```python
from build123d import *

# Parameters (mm, degrees)
SKETCH1_W           = 16.5
SKETCH1_H           = 11.5
SKETCH1_W_2         = 10.5
SKETCH1_H_2         = 5.5
BOSS_EXTRUDE1_DEPTH = 17
CUT_EXTRUDE1_REACH  = 28.334
SKETCH2_R           = 2.5
SKETCH3_W           = 16.5
SKETCH3_H           = 11.5
BOSS_EXTRUDE2_DEPTH = 3
BOSS_EXTRUDE3_START = -11
SKETCH4_W           = 21.75
SKETCH4_H           = 11
BOSS_EXTRUDE3_DEPTH = 4
CHAMFER1_SIZE       = 5
CHAMFER2_SIZE       = 3
SKETCH5_R           = 1.1
SKETCH5_W           = 3
SKETCH5_H           = 2.684
BOSS_EXTRUDE4_DEPTH = 7
BOSS_EXTRUDE5_DEPTH = 11
CUT_EXTRUDE2_REACH  = 41.144
SKETCH7_W           = 10.5
SKETCH7_H           = 1.5


with BuildPart() as part:
    # Sketch1 → Boss-Extrude1 (new body)
    with BuildSketch(Plane(origin=(0, 0, 0), x_dir=(1, 0, 0), z_dir=(0, 1, 0))):
        with Locations((8.25, 5.75)):
            Rectangle(SKETCH1_W, SKETCH1_H)
        with Locations((8.25, 5.75)):
            Rectangle(SKETCH1_W_2, SKETCH1_H_2, mode=Mode.SUBTRACT)
    extrude(amount=BOSS_EXTRUDE1_DEPTH)

    # Sketch2 → Cut-Extrude1 (cut, up to next)
    with BuildSketch(Plane(origin=(0, 0, -11.5), x_dir=(-1, 0, 0), z_dir=(0, 0, -1)), mode=Mode.PRIVATE) as cut_extrude1_sk1:
        with Locations((-8.25, 10.5)):
            Circle(SKETCH2_R)
    cut_extrude1_tool1 = extrude(cut_extrude1_sk1.sketch, amount=-CUT_EXTRUDE1_REACH, mode=Mode.PRIVATE) & part.part
    add(cut_extrude1_tool1.solids().sort_by_distance((8.25, 10.5, -11.5))[0], mode=Mode.SUBTRACT)

    # Sketch3 → Boss-Extrude2 (add)
    with BuildSketch(Plane(origin=(0, 17, 0), x_dir=(1, 0, 0), z_dir=(0, 1, 0))):
        with Locations((8.25, 5.75)):
            Rectangle(SKETCH3_W, SKETCH3_H)
    extrude(amount=BOSS_EXTRUDE2_DEPTH)

    # Sketch4 → Boss-Extrude3 (add)
    with BuildSketch(Plane(origin=(0, 20, 0), x_dir=(1, 0, 0), z_dir=(0, 1, 0)).offset(BOSS_EXTRUDE3_START)):
        with Locations((-10.875, -2.176)):
            Rectangle(SKETCH4_W, SKETCH4_H)
    extrude(amount=BOSS_EXTRUDE3_DEPTH)

    # Chamfer1
    chamfer1_edges = [part.edges().sort_by_distance(p)[0] for p in [
        (0, 11, 0),
        (0, 11, -3.324),
    ]]
    chamfer(chamfer1_edges, length=CHAMFER1_SIZE)

    # Chamfer2
    chamfer2_edges = [part.edges().sort_by_distance(p)[0] for p in [
        (0, 13, -4.162),
        (0, 9, -4.162),
        (2.5, 13, 0),
        (2.5, 9, 0),
    ]]
    chamfer(chamfer2_edges, length=CHAMFER2_SIZE)

    # Sketch5 → Boss-Extrude4 (add)
    with BuildSketch(Plane(origin=(0, 13, 0), x_dir=(1, 0, 0), z_dir=(0, 1, 0))):
        with Locations(Location((-19.15, -2.46, 0), (0, 0, 270))):
            Circle(SKETCH5_R)
        with Locations(Location((-9.5, -2.46, 0), (0, 0, 270))):
            Circle(SKETCH5_R)
        with Locations((-19.15, 1.982)):
            Rectangle(SKETCH5_W, SKETCH5_H)
        with Locations((-9.5, 1.982)):
            Rectangle(SKETCH5_W, SKETCH5_H)
    extrude(amount=BOSS_EXTRUDE4_DEPTH)

    # Sketch6 → Boss-Extrude5 (add)
    with BuildSketch(Plane.XY.offset(7.676)):
        Polygon((-21.75, 13), (-24.65, 13), (-24.65, 20), (-27.65, 20), (-27.65, 9), (-21.75, 9), align=None)
    extrude(amount=-BOSS_EXTRUDE5_DEPTH)

    # Sketch7 → Cut-Extrude2 (cut, up to next)
    with BuildSketch(Plane(origin=(0, 0, -11.5), x_dir=(-1, 0, 0), z_dir=(0, 0, -1)), mode=Mode.PRIVATE) as cut_extrude2_sk1:
        with Locations((-8.25, 16.25)):
            Rectangle(SKETCH7_W, SKETCH7_H)
    cut_extrude2_tool1 = extrude(cut_extrude2_sk1.sketch, amount=-CUT_EXTRUDE2_REACH, mode=Mode.PRIVATE) & part.part
    add(cut_extrude2_tool1.solids().sort_by_distance((8.25, 16.25, -11.5))[0], mode=Mode.SUBTRACT)


solid = part.part
```
The listing builds one solid part. Answer for the finished solid, in the listing's coordinates (mm). A direction names the side the tool comes from. Give positions to 0.01 mm unless a question says otherwise; leave off trailing zeros. Order: outer loops, then holes, each group sorted by start corner. A loop starts at its lowest first (then second) coordinate and runs counter-clockwise, first axis right, second up. Notation, with made-up numbers: (14.25, -35) -> (62.25, -35) arc R31 ccw to (62.25, -8) -> close; hole circle Ø5 at (-34.5, 39.25). An arc over 180 degrees is marked (long way). Answer as a JSON object with one key per item and string values. Group by question number.
Item 1: A tool of negligible diameter and unlimited length cuts with its end or side. For faces 1 (the flat face through (-17, 12, 7.676)), 2 (the cylindrical face through (-10.17, 16.45, 1.59)), 3 (the flat face through (1, 15, 1)), 4 (the flat face through (-20.65, 16, -2)), from which of +Z, -Z, +X, -X, +Y, -Y can it reach the whole face along a straight path? Write none if from no direction.
Item 2: Determine the mould class of faces 5 (the cylindrical face through (8.79, 8.06, -10.02)), 6 (the flat face through (8, 8, -3)), 7 (the flat face through (8, 17, -7)), 8 (the flat face through (1, 8, 2)) for opening direction Y: pulls with the +Y half, pulls with the -Y half, needs draft (parallel to the pull), parting line crosses it, or undercut.
Item 3: The part is cut by section B-B on x = 8.25. Write down the section's boundary in (y, z), and give its area (3 significant figures).
Item 4: The part is cut by section A-A on y = 10.5. Write down the section's boundary in (x, z).
Item 5: Consider L1, parallel to Y at x = 8.25, z = -10.55; L2, parallel to X at y = 3.5, z = -3.5; L3, parallel to Z at x = 9.5, y = 1.5. Determine where each line is inside the solid, lowest interval first. Write a range as from..to.
Item 6: Flat-ended cylindrical pins translate along their axes: pin 1 (10 mm diameter, centred on x = -15.5, y = 12.5, fed in from -Z); pin 2 (8 mm diameter, centred on x = 11, z = -9, fed in from -Y); pin 3 (3 mm diameter, centred on x = -14.5, y = 17, fed in from +Z); pin 4 (2.5 mm diameter, centred on x = -9, y = 17.5, fed in from +Z). Find the tip coordinate at first contact, or state that the pin passes through.
Item 7: The part is cut by section C-C on x = -9.5. Write down the section's boundary in (y, z).
Item 8: The part is cut by section D-D on z = 2.46. Write down the section's boundary in (x, y).
Result set:
{
 "1": {"face 1": "+Z, +X, -X, +Y, -Y", "face 2": "+Y", "face 3": "+Z, +X, +Y", "face 4": "+Z, -Z, +Y"},
 "2": {"face 5": "undercut", "face 6": "needs draft", "face 7": "undercut", "face 8": "pulls with the -Y half"},
 "3": {"outline": "(0, -11.5) -> (8, -11.5) -> (8, -8.5) -> (0, -8.5) -> close; (0, -3) -> (17, -3) -> (17, -11.5) -> (20, -11.5) -> (20, 0) -> (0, 0) -> close; (13, -11.5) -> (15.5, -11.5) -> (15.5, -8.5) -> (13, -8.5) -> close", "area": "117 mm²"},
 "4": {"outline": "(-27.65, -3.32) -> (-5, -3.32) -> (0, -8.32) -> (0, -11.5) -> (5.75, -11.5) -> (5.75, -8.5) -> (3, -8.5) -> (3, -3) -> (13.5, -3) -> (13.5, -8.5) -> (10.75, -8.5) -> (10.75, -11.5) -> (16.5, -11.5) -> (16.5, 0) -> (5, 0) -> (0, 5) -> (0, 7.68) -> (-27.65, 7.68) -> close"},
 "5": {"L1": "0..8, 13..15.5, 17..20", "L2": "0..3, 13.5..16.5", "L3": "-11.5..-8.5, -3..0"},
 "6": {"pin 1": "z = -3.32", "pin 2": "y = 0", "pin 3": "through", "pin 4": "z = 3.56"},
 "7": {"outline": "(9, -3.32) -> (20, -3.32) -> (20, -0.64) -> (13, -0.64) -> (13, 1.36) -> (20, 1.36) -> (20, 3.56) -> (13, 3.56) -> (13, 7.68) -> (9, 7.68) -> close"},
 "8": {"outline": "(-27.65, 9) -> (-3, 9) -> (-2.46, 8.46) -> (2.54, 8.46) -> (2.54, 13.54) -> (-2.46, 13.54) -> (-3, 13) -> (-8.4, 13) -> (-8.4, 20) -> (-10.6, 20) -> (-10.6, 13) -> (-18.05, 13) -> (-18.05, 20) -> (-20.25, 20) -> (-20.25, 13) -> (-24.65, 13) -> (-24.65, 20) -> (-27.65, 20) -> close"}
}
